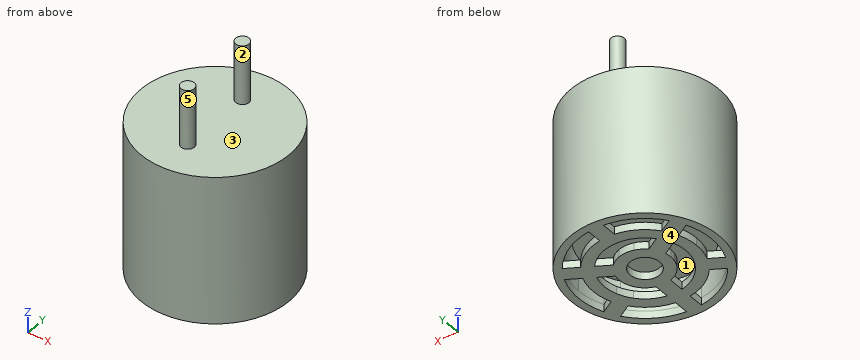
from build123d import *
from build123d.topology import SkipClean

# Parameters (mm, degrees)
SKETCH1_R           = 5
BOSS_EXTRUDE1_DEPTH = 10
SKETCH2_R           = 0.45
BOSS_EXTRUDE2_DEPTH = 4
SHELL1_START        = 0.5
SHELL1_OUTLINE_R    = 4.5
SHELL1_DEPTH        = 8.5
SKETCH4_R           = 1
CUT_EXTRUDE2_DEPTH  = 4
SKETCH5_R           = 4
BOSS_EXTRUDE3_DEPTH = 7


# Read off the part's stored shape, not the designer's step: Shell1
with BuildPart() as part:
    # Sketch1 → Boss-Extrude1 (new body)
    with BuildSketch(Plane.XY):
        Circle(SKETCH1_R)
    extrude(amount=BOSS_EXTRUDE1_DEPTH)

    # Sketch2 → Boss-Extrude2 (add)
    with BuildSketch(Plane.XY.offset(10)):
        with Locations((0, 2.5)):
            Circle(SKETCH2_R)
        with Locations((0, -2.5)):
            Circle(SKETCH2_R)
    extrude(amount=BOSS_EXTRUDE2_DEPTH)

    # Shell1 outline → Shell1 (cut)
    with BuildSketch(Plane.XY.offset(SHELL1_START)):
        Circle(SHELL1_OUTLINE_R)
    extrude(amount=SHELL1_DEPTH, mode=Mode.SUBTRACT)

    # Sketch4 → Cut-Extrude2 (cut)
    with SkipClean():  # the faces are left unmerged after this step: merging them gives an invalid solid
        with BuildSketch(Plane(origin=(0, 0, 0), x_dir=(-1, 0, 0), z_dir=(0, 0, -1))):
            with BuildLine():
                ThreePointArc((-2.75, 2.165063509), (-1.75, 3.031088913), (-0.5, 3.464101615))
                Line((-0.5, 3.464101615), (-0.5, 4.472135955))
                ThreePointArc((-0.5, 4.472135955), (-2.25, 3.897114317), (-3.622983346, 2.669080679))
                Line((-3.622983346, 2.669080679), (-2.75, 2.165063509))
            make_face()
            with BuildLine():
                ThreePointArc((0.5, 3.464101615), (1.75, 3.031088913), (2.75, 2.165063509))
                Line((2.75, 2.165063509), (3.622983346, 2.669080679))
                ThreePointArc((3.622983346, 2.669080679), (2.25, 3.897114317), (0.5, 4.472135955))
                Line((0.5, 4.472135955), (0.5, 3.464101615))
            make_face()
            with BuildLine():
                ThreePointArc((0.5, 1.677050983), (0.875, 1.515544457), (1.202368755, 1.271538193))
                Line((1.202368755, 1.271538193), (2.091874249, 1.78509443))
                ThreePointArc((2.091874249, 1.78509443), (1.375, 2.38156986), (0.5, 2.704163457))
                Line((0.5, 2.704163457), (0.5, 1.677050983))
            make_face()
            with BuildLine():
                ThreePointArc((-1.202368755, 1.271538193), (-0.875, 1.515544457), (-0.5, 1.677050983))
                Line((-0.5, 1.677050983), (-0.5, 2.704163457))
                ThreePointArc((-0.5, 2.704163457), (-1.375, 2.38156986), (-2.091874249, 1.78509443))
                Line((-2.091874249, 1.78509443), (-1.202368755, 1.271538193))
            make_face()
            Circle(SKETCH4_R)
            with BuildLine():
                ThreePointArc((-1.702368755, -0.40551279), (-1.75, 0), (-1.702368755, 0.40551279))
                Line((-1.702368755, 0.40551279), (-2.591874249, 0.919069026))
                ThreePointArc((-2.591874249, 0.919069026), (-2.75, 0), (-2.591874249, -0.919069026))
                Line((-2.591874249, -0.919069026), (-1.702368755, -0.40551279))
            make_face()
            with BuildLine():
                Line((-0.5, -2.704163457), (-0.5, -1.677050983))
                ThreePointArc((-0.5, -1.677050983), (-0.875, -1.515544457), (-1.202368755, -1.271538193))
                Line((-1.202368755, -1.271538193), (-2.091874249, -1.78509443))
                ThreePointArc((-2.091874249, -1.78509443), (-1.375, -2.38156986), (-0.5, -2.704163457))
            make_face()
            with BuildLine():
                Line((2.091874249, -1.78509443), (1.202368755, -1.271538193))
                ThreePointArc((1.202368755, -1.271538193), (0.875, -1.515544457), (0.5, -1.677050983))
                Line((0.5, -1.677050983), (0.5, -2.704163457))
                ThreePointArc((0.5, -2.704163457), (1.375, -2.38156986), (2.091874249, -1.78509443))
            make_face()
            with BuildLine():
                Line((2.591874249, 0.919069026), (1.702368755, 0.40551279))
                ThreePointArc((1.702368755, 0.40551279), (1.738051398, 0.204150287), (1.75, 0))
                ThreePointArc((1.75, 0), (1.738051398, -0.204150287), (1.702368755, -0.40551279))
                Line((1.702368755, -0.40551279), (2.591874249, -0.919069026))
                ThreePointArc((2.591874249, -0.919069026), (2.710180269, -0.466286293), (2.75, 0))
                ThreePointArc((2.75, 0), (2.710180269, 0.466286293), (2.591874249, 0.919069026))
            make_face()
            with BuildLine():
                Line((2.591874249, -0.919069026), (1.702368755, -0.40551279))
                ThreePointArc((1.702368755, -0.40551279), (1.515544457, -0.875), (1.202368755, -1.271538193))
                Line((1.202368755, -1.271538193), (2.091874249, -1.78509443))
                ThreePointArc((2.091874249, -1.78509443), (2.38156986, -1.375), (2.591874249, -0.919069026))
            make_face()
            with BuildLine():
                ThreePointArc((-1.202368755, -1.271538193), (-1.515544457, -0.875), (-1.702368755, -0.40551279))
                Line((-1.702368755, -0.40551279), (-2.591874249, -0.919069026))
                ThreePointArc((-2.591874249, -0.919069026), (-2.38156986, -1.375), (-2.091874249, -1.78509443))
                Line((-2.091874249, -1.78509443), (-1.202368755, -1.271538193))
            make_face()
            with BuildLine():
                ThreePointArc((-0.5, 1.677050983), (0, 1.75), (0.5, 1.677050983))
                Line((0.5, 1.677050983), (0.5, 2.704163457))
                ThreePointArc((0.5, 2.704163457), (0, 2.75), (-0.5, 2.704163457))
                Line((-0.5, 2.704163457), (-0.5, 1.677050983))
            make_face()
            with BuildLine():
                Line((4.122983346, 1.803055276), (3.25, 1.299038106))
                ThreePointArc((3.25, 1.299038106), (3.436931771, 0.661437828), (3.5, 0))
                ThreePointArc((3.5, 0), (3.436931771, -0.661437828), (3.25, -1.299038106))
                Line((3.25, -1.299038106), (4.122983346, -1.803055276))
                ThreePointArc((4.122983346, -1.803055276), (4.40473751, -0.921025228), (4.5, 0))
                ThreePointArc((4.5, 0), (4.40473751, 0.921025228), (4.122983346, 1.803055276))
            make_face()
            with BuildLine():
                Line((3.622983346, -2.669080679), (2.75, -2.165063509))
                ThreePointArc((2.75, -2.165063509), (1.75, -3.031088913), (0.5, -3.464101615))
                Line((0.5, -3.464101615), (0.5, -4.472135955))
                ThreePointArc((0.5, -4.472135955), (2.25, -3.897114317), (3.622983346, -2.669080679))
            make_face()
            with BuildLine():
                Line((-0.5, -4.472135955), (-0.5, -3.464101615))
                ThreePointArc((-0.5, -3.464101615), (-1.75, -3.031088913), (-2.75, -2.165063509))
                Line((-2.75, -2.165063509), (-3.622983346, -2.669080679))
                ThreePointArc((-3.622983346, -2.669080679), (-2.25, -3.897114317), (-0.5, -4.472135955))
            make_face()
            with BuildLine():
                ThreePointArc((-3.25, -1.299038106), (-3.5, 0), (-3.25, 1.299038106))
                Line((-3.25, 1.299038106), (-4.122983346, 1.803055276))
                ThreePointArc((-4.122983346, 1.803055276), (-4.5, 0), (-4.122983346, -1.803055276))
                Line((-4.122983346, -1.803055276), (-3.25, -1.299038106))
            make_face()
        extrude(amount=-CUT_EXTRUDE2_DEPTH, mode=Mode.SUBTRACT)

    # Sketch5 → Boss-Extrude3 (add)
    with SkipClean():  # the faces are left unmerged after this step: merging them gives an invalid solid
        with BuildSketch(Plane(origin=(0, 0, 9), x_dir=(-1, 0, 0), z_dir=(0, 0, -1))):
            with Locations(Location((0, 0, 0), (0, 0, 180))):
                Circle(SKETCH5_R)
        extrude(amount=BOSS_EXTRUDE3_DEPTH)


solid = part.part
Read the model definition and answer for the solid it produces. Units are mm, in the model's axes. Face numbers are marked on the shaded views. A direction names the side the tool comes from. Round coordinates to 2 decimals unless told otherwise and drop trailing zeros. Order: outer loops, then holes, each group sorted by start corner. A loop starts at its lowest first (then second) coordinate and runs counter-clockwise, first axis right, second up.
1) The part is cut by section B-B on z = 8.5. Write down the section's boundary in (x, y), plus the area to 3 significant figures.
2) The part is cut by section A-A on x = 0. Write down the section's boundary in (y, z), plus the area to 3 significant figures.
3) Straight lines are drawn through the part: L1, parallel to Y at x = 0, z = 4.5; L2, parallel to Y at x = 0, z = 0.2; L3, parallel to X at y = -1.25, z = 5.75. For each, find the intervals that lie inside material, in ascending order.
4) For the marked faces 4 and 5, determine the directions among +Z, -Z, +X, -X, +Y, -Y from which every point of the face is accessible in a straight line to the end or side of a thin tool.
5) The mould has two halves that part along X. Classify the marked faces 1, 2 and 3: released by +X, released by -X, zero draft, split by the parting line, or undercut.
6) The part is cut by section C-C on z = 1.75. Write down the section's boundary in (x, y).
7) The part is cut by section D-D on y = -2.5. Give the number of separate pieces and of enclosed holes in the cut face, plus the area to 3 significant figures.
8) Flat-ended cylindrical pins translate along their axes: pin 1 (1.2 mm diameter, centred on x = 0, y = 0, fed in from +Z); pin 2 (1 mm diameter, centred on x = -1, z = 7, fed in from +Y). Find the tip coordinate at first contact, or state that the pin passes through.
Resolved:
1. outline: circle Ø10 at (0, 0); circle Ø8 at (0, 0); hole circle Ø9 at (0, 0)
1. area: 65.2 mm2
2. outline: (-5, 0) - (-1, 0) - (-1, 0.5) - (-4.5, 0.5) - (-4.5, 9) - (-4, 9) - (-4, 2) - (4, 2) - (4, 9) - (4.5, 9) - (4.5, 0.5) - (2.75, 0.5) - (2.75, 0) - (5, 0) - (5, 10) - (2.95, 10) - (2.95, 14) - (2.05, 14) - (2.05, 10) - (-2.05, 10) - (-2.05, 14) - (-2.95, 14) - (-2.95, 10) - (-5, 10) - close; (1, 0) - (1.75, 0) - (1.75, 0.5) - (1, 0.5) - close
2. area: 85.2 mm2
3. L1: y = -5 to -4.5, -4 to 4, 4.5 to 5
3. L2: y = -5 to -1, 1 to 1.75, 2.75 to 5
3. L3: x = -4.84 to -4.32, -3.8 to 3.8, 4.32 to 4.84
4. face 4: -Z, +X, -X, +Y, -Y
4. face 5: +Z
5. face 1: undercut
5. face 2: split by the parting line
5. face 3: zero draft
6. outline: circle Ø10 at (0, 0); hole circle Ø9 at (0, 0)
7. separate pieces: 4
7. enclosed holes: 0
7. area: 68.8 mm2
8. pin 1: stops at z = 10
8. pin 2: stops at y = 4.97
